Check sheet for the modelled part. Datum: model origin and axes. Units: mm. Face numbers are marked on the shaded views. Coordinates: 2 decimals unless noted, no trailing zeros. Write each loop counter-clockwise with the first axis right and the second up, starting at its lowest first coordinate (ties: lowest second). Pieces come first, ordered by that corner, then holes. Notation, with made-up numbers: M 57.25,-21.5 L 72.25,-21.5 A16 ccw 72.25,1.5 Z; hole C 51.25,13 d9. An arc over 180 degrees is marked long. Answer as CSV lines item,"result". Start each with the question number.
Q1. Sectioned sample at D-D, the plane y = 2. Record the cut outline in (x, z).
Q2. Thickness scan on line 1 along X through (y, z) = (1.95, 0); line 2 along X through (y, z) = (2.25, -18); line 3 along X through (y, z) = (5.75, 0). Record the ranges inside material, lowest first. Write a range as from..to.
Q3. Sectioned sample at B-B, the plane z = 0. Record the cut outline in (x, y).
Q4. Depth check by flat-ended pin: pin 1 Ø5 at (x, z) = (20.28, 20.28) entering from -Y; pin 2 Ø6 at (x, z) = (20.28, -20.28) entering from -Y. Enter the tip coordinate at first touch or a pass-through.
Q5. Sectioned sample at A-A, the plane x = 0. Record the cut outline in (y, z).
Q6. Sectioned sample at C-C, the plane x = -21. Record the cut outline in (y, z).
Q7. Mould release check, pull along Z, two halves, no side actions. Record for the marked faces 1, 2, 3 and 4: pulls with the +Z half, pulls with the -Z half, needs draft (parallel to the pull), parting line crosses it, or undercut.
from build123d import *

# Parameters (mm, degrees)
SKETCH1_W           = 50
SKETCH1_H           = 50
SKETCH1_R           = 12
BOSS_EXTRUDE1_DEPTH = 3
SKETCH2_W           = 50
SKETCH2_H           = 50
SKETCH2_R           = 22
BOSS_EXTRUDE2_DEPTH = 6
SKETCH3_R           = 2.65
CUT_EXTRUDE1_DEPTH  = 30


with BuildPart() as part:
    # Sketch1 → Boss-Extrude1 (new body)
    with BuildSketch(Plane(origin=(0, 0, 0), x_dir=(1, 0, 0), z_dir=(0, 1, 0))):
        Rectangle(SKETCH1_W, SKETCH1_H)
        with Locations(Location((0, 0, 0), (0, 0, 270))):
            Circle(SKETCH1_R, mode=Mode.SUBTRACT)
    extrude(amount=BOSS_EXTRUDE1_DEPTH)

    # Sketch2 → Boss-Extrude2 (add)
    with BuildSketch(Plane(origin=(0, 3, 0), x_dir=(1, 0, 0), z_dir=(0, 1, 0))):
        Rectangle(SKETCH2_W, SKETCH2_H)
        with Locations(Location((0, 0, 0), (0, 0, 270))):
            Circle(SKETCH2_R, mode=Mode.SUBTRACT)
    extrude(amount=BOSS_EXTRUDE2_DEPTH)

    # Sketch3 → Cut-Extrude1 (cut)
    with BuildSketch(Plane(origin=(0, 9, 0), x_dir=(1, 0, 0), z_dir=(0, 1, 0))):
        with Locations(Location((-20.278174593, 20.278174593, 0), (0, 0, 270))):
            Circle(SKETCH3_R)
        with Locations(Location((-20.278174593, -20.278174593, 0), (0, 0, 90))):
            Circle(SKETCH3_R)
        with Locations(Location((20.278174593, -20.278174593, 0), (0, 0, 270))):
            Circle(SKETCH3_R)
        with Locations(Location((20.278174593, 20.278174593, 0), (0, 0, 90))):
            Circle(SKETCH3_R)
    extrude(amount=-CUT_EXTRUDE1_DEPTH, mode=Mode.SUBTRACT)


solid = part.part
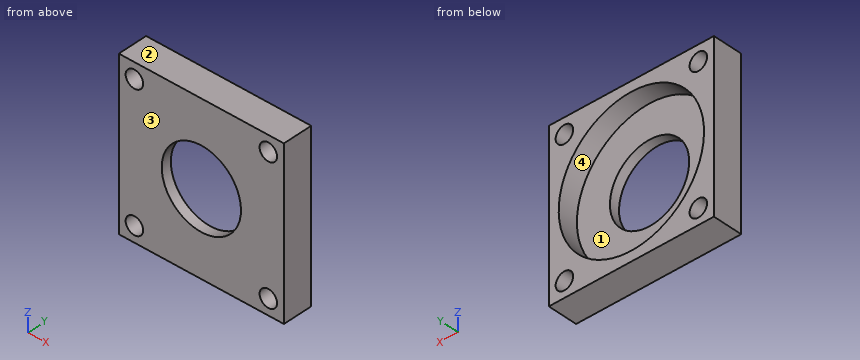
Output:
1,outline,"M -25,-25 L 25,-25 L 25,25 L -25,25 Z; hole C -20.28,-20.28 d5.3; hole C -20.28,20.28 d5.3; hole C 0,0 d24; hole C 20.28,-20.28 d5.3; hole C 20.28,20.28 d5.3"
2,line 1,"x = -25..-12, 12..25"
2,line 2,"x = -25..-21.63, -18.92..18.92, 21.63..25"
2,line 3,"x = -25..-22, 22..25"
3,outline,"M -25,0 L -12,0 L -12,3 L -22,3 L -22,9 L -25,9 Z; M 12,0 L 25,0 L 25,9 L 22,9 L 22,3 L 12,3 Z"
4,pin 1,"passes through"
4,pin 2,"stops at y = 0"
5,outline,"M 0,-25 L 9,-25 L 9,-22 L 3,-22 L 3,-12 L 0,-12 Z; M 0,12 L 3,12 L 3,22 L 9,22 L 9,25 L 0,25 Z"
6,outline,"M 0,-25 L 9,-25 L 9,-22.83 L 0,-22.83 Z; M 0,-17.73 L 9,-17.73 L 9,-6.56 L 3,-6.56 L 3,6.56 L 9,6.56 L 9,17.73 L 0,17.73 Z; M 0,22.83 L 9,22.83 L 9,25 L 0,25 Z"
7,face 1,"undercut"
7,face 2,"pulls with the +Z half"
7,face 3,"needs draft"
7,face 4,"undercut"
